from build123d import *

# Parameters (mm, degrees)
BOSS_EXTRUDE1_DEPTH = 5
SKETCH2_W           = 35
SKETCH2_H           = 65
CUT_EXTRUDE1_DEPTH  = 10
CUT_EXTRUDE2_DEPTH  = 5
SKETCH4_W           = 30
SKETCH4_H           = 5
BOSS_EXTRUDE2_DEPTH = 5
SKETCH5_W           = 20
SKETCH5_H           = 5
CUT_EXTRUDE3_DEPTH  = 5
SKETCH6_R           = 2.1
CUT_EXTRUDE4_DEPTH  = 5
BOSS_EXTRUDE3_DEPTH = 5
SKETCH8_W           = 4.2
SKETCH8_H           = 5
SKETCH8_W_2         = 10
SKETCH8_H_2         = 10
CUT_EXTRUDE5_DEPTH  = 5
SKETCH9_W           = 10
SKETCH9_H           = 3
CUT_EXTRUDE6_DEPTH  = 10


with BuildPart() as part:
    # Sketch1 → Boss-Extrude1 (new body)
    with BuildSketch(Plane.XY):
        Polygon((95, -5), (95, 0), (115, 0), (115, 15), (120, 15), (120, 40), (115, 40), (115, 55), (100, 55), (100, 60), (70, 60), (70, 55), (-70, 55), (-70, 60), (-100, 60), (-100, 55), (-115, 55), (-115, 40), (-120, 40), (-120, 15), (-115, 15), (-115, 0), (-95, 0), (-95, -5), (-35, -5), (-35, 0), (35, 0), (35, -5), align=None)
    extrude(amount=BOSS_EXTRUDE1_DEPTH)

    # Sketch2 → Cut-Extrude1 (cut)
    with BuildSketch(Plane(origin=(0, 0, 0), x_dir=(-1, 0, 0), z_dir=(0, 0, -1))):
        with Locations((102.5, 27.5)):
            Rectangle(SKETCH2_W, SKETCH2_H)
        with Locations((-102.5, 27.5)):
            Rectangle(SKETCH2_W, SKETCH2_H)
    extrude(amount=-CUT_EXTRUDE1_DEPTH, mode=Mode.SUBTRACT)

    # Sketch3 → Cut-Extrude2 (cut)
    with BuildSketch(Plane(origin=(0, 0, 0), x_dir=(-1, 0, 0), z_dir=(0, 0, -1))):
        with BuildLine():
            Line((58.770676698, 55), (51.229323302, 55))
            ThreePointArc((51.229323302, 55), (55, 53.28359517), (58.770676698, 55))
        make_face()
        with BuildLine():
            Line((-58.770676698, 55), (-51.229323302, 55))
            ThreePointArc((-51.229323302, 55), (-55, 53.28359517), (-58.770676698, 55))
        make_face()
    extrude(amount=-CUT_EXTRUDE2_DEPTH, mode=Mode.SUBTRACT)

    # Sketch4 → Boss-Extrude2 (add)
    with BuildSketch(Plane(origin=(0, 55, 0), x_dir=(1, 0, 0), z_dir=(0, 1, 0))):
        with Locations((0, -2.5)):
            Rectangle(SKETCH4_W, SKETCH4_H)
    extrude(amount=BOSS_EXTRUDE2_DEPTH)

    # Sketch5 → Cut-Extrude3 (cut)
    with BuildSketch(Plane(origin=(0, 0, 0), x_dir=(-1, 0, 0), z_dir=(0, 0, -1))):
        with Locations((-69.8, -2.5)):
            Rectangle(SKETCH5_W, SKETCH5_H)
        with Locations((69.8, -2.5)):
            Rectangle(SKETCH5_W, SKETCH5_H)
    extrude(amount=-CUT_EXTRUDE3_DEPTH, mode=Mode.SUBTRACT)

    # Sketch6 → Cut-Extrude4 (cut)
    with BuildSketch(Plane(origin=(0, 0, 0), x_dir=(-1, 0, 0), z_dir=(0, 0, -1))):
        with Locations((0, 57.5)):
            Circle(SKETCH6_R)
    extrude(amount=-CUT_EXTRUDE4_DEPTH, mode=Mode.SUBTRACT)

    # Sketch7 → Boss-Extrude3 (add)
    with BuildSketch(Plane(origin=(0, 0, 0), x_dir=(-1, 0, 0), z_dir=(0, 0, -1))):
        with BuildLine():
            Line((4.330127019, 60), (-4.330127019, 60))
            ThreePointArc((-4.330127019, 60), (0, 62.5), (4.330127019, 60))
        make_face()
    extrude(amount=-BOSS_EXTRUDE3_DEPTH)

    # Sketch8 → Cut-Extrude5 (cut)
    with BuildSketch(Plane(origin=(0, 0, 0), x_dir=(-1, 0, 0), z_dir=(0, 0, -1))):
        with Locations((69.8, 2.5)):
            Rectangle(SKETCH8_W, SKETCH8_H)
        with Locations((69.8, 10)):
            Rectangle(SKETCH8_W_2, SKETCH8_H_2)
        with Locations((-69.8, 10)):
            Rectangle(SKETCH8_W_2, SKETCH8_H_2)
        with Locations((-69.8, 2.5)):
            Rectangle(SKETCH8_W, SKETCH8_H)
        with Locations((0, 2.5)):
            Rectangle(SKETCH8_W, SKETCH8_H)
        with Locations((0, 10)):
            Rectangle(SKETCH8_W_2, SKETCH8_H_2)
    extrude(amount=-CUT_EXTRUDE5_DEPTH, mode=Mode.SUBTRACT)

    # Sketch9 → Cut-Extrude6 (cut)
    with BuildSketch(Plane(origin=(0, 0, 0), x_dir=(-1, 0, 0), z_dir=(0, 0, -1))):
        with Locations((-25.5, 27.625214192)):
            Rectangle(SKETCH9_W, SKETCH9_H)
        with Locations((25.5, 27.625214192)):
            Rectangle(SKETCH9_W, SKETCH9_H)
    extrude(amount=-CUT_EXTRUDE6_DEPTH, mode=Mode.SUBTRACT)


solid = part.part
Geometry check sheet. Reference: the model listing, model coordinates, mm. A direction names the side the tool comes from. Round coordinates to 2 decimals unless told otherwise and drop trailing zeros. Write each loop counter-clockwise with the first axis right and the second up, starting at its lowest first coordinate (ties: lowest second). Pieces come first, ordered by that corner, then holes.
Item 1: Section check A-A (x = 0). Record the boundary of the cut face in (y, z).
Determined:
outline: (15, 0) - (55.4, 0) - (55.4, 5) - (15, 5) - close; (59.6, 0) - (62.5, 0) - (62.5, 5) - (59.6, 5) - close
Item 2: Go/stop test with flat-tipped pins: pin 1 Ø1.5 at (x, z) = (66.5, 2.5) entering from +Y; pin 2 Ø2.5 at (x, z) = (4, 2.5) entering from +Y; pin 3 Ø0.9 at (x, z) = (-72.5, 2.5) entering from +Y; pin 4 Ø10 at (x, y) = (64, 54.5) entering from -Z. Record where each tip stops, or that it passes through.
Determined:
pin 1: stops at y = 55
pin 2: stops at y = 61.68
pin 3: stops at y = 60
pin 4: stops at z = 0
Item 3: Material ranges on line 1 along X through (y, z) = (9, 3); line 2 along X through (y, z) = (29, 1.4); line 3 along Y through (x, z) = (0, 3.35), recorded low to high.
Determined:
line 1: x = -85 to -74.8, -64.8 to -5, 5 to 64.8, 74.8 to 85
line 2: x = -85 to -30.5, -20.5 to 20.5, 30.5 to 85
line 3: y = 15 to 55.4, 59.6 to 62.5
Item 4: Access from +Z, -Z, +X, -X, +Y, -Y to the whole of each face (thin tool, end or side, straight path). Record for faces 5 (the face through (76, 0, 2)), 6 (the face through (33, 55, 2)), 7 (the face through (64.8, 10, 2)).
Determined:
face 5: +Z, -Z, -Y
face 6: +Z, -Z, +Y
face 7: +Z, -Z
Item 5: Section check B-B (y = 57.5). Record the boundary of the cut face in (x, z).
Determined:
outline: (-85, 0) - (-70, 0) - (-70, 5) - (-85, 5) - close; (-15, 0) - (-2.1, 0) - (-2.1, 5) - (-15, 5) - close; (2.1, 0) - (15, 0) - (15, 5) - (2.1, 5) - close; (70, 0) - (85, 0) - (85, 5) - (70, 5) - close
Item 6: Section check C-C (x = -24). Record the boundary of the cut face in (y, z).
Determined:
outline: (0, 0) - (26.13, 0) - (26.13, 5) - (0, 5) - close; (29.13, 0) - (55, 0) - (55, 5) - (29.13, 5) - close
Item 7: Section check D-D (z = 2.5). Give the number of separate pieces and of enclosed holes in the cut face, plus the area to 3 significant figures.
Determined:
separate pieces: 1
enclosed holes: 3
area: 9,510 mm2
Item 8: Mould release check, pull along Y, two halves, no side actions. Record for faces 1 (the face through (85, 27, 2)), 2 (the face through (-33, 55, 2)), 3 (the face through (0.46, 55.45, 2.46)), 4 (the face through (-4, 5, 2)): +Y half, -Y half, draft (parallel to the pull), parting line (faces both ways), or undercut.
Determined:
face 1: draft
face 2: +Y half
face 3: undercut
face 4: undercut
